For this review, take the finished solid that the model builds, in its own axes (mm). Face numbers are marked on the shaded views. Give positions to 0.01 mm unless a question says otherwise; leave off trailing zeros. Loops run counter-clockwise (first coordinate to the right, second up) from the corner with the lowest first, then second, coordinate; pieces in that order, holes last. Notation, with made-up numbers: (-3.75, -38) - (30.25, -38) arc R23 cw to (30.25, -9) - close; hole circle Ø10 at (44.25, 7). An arc over 180 degrees is marked (long way). Put each result on its own line as item: value. Start each with the question number.
from build123d import *

# Parameters (mm, degrees)
F2_R     = 2.9212519553
F3_DEPTH = 25


# Not quite as in the source:
# - a fillet or chamfer that OpenCascade refuses, or shapes differently, is made with other operations: its cross-section is extruded or revolved along the edge and cut away or added


with BuildPart() as f1:
    # F0 (on Front) → F1 (revolve)
    with BuildSketch(Plane.XZ):
        Polygon((0, 18.8674032688), (0, 15.0357997045), (10, 15.0357997045), (10, 18.8674032688), (6.7462138832, 18.8674032688), (6.7462138832, 29.4962655753), (17.0517656952, 29.4962655753), (17.0517656952, 34.9722243845), (0, 34.9722243845), (0, 29.4962655753), (2.411958063, 29.4962655753), (2.411958063, 18.8674032688), align=None)
    revolve(axis=Axis((6.3371746801, 0, 0), (1, 0, 0)))

    # F2 (on face) → F3 (cut)
    with BuildSketch(Plane(origin=(2.411958063, 0, 0), x_dir=(0, -1, 0), z_dir=(-1, 0, 0))):
        with Locations((-22.6866142127, 7.3713277985)):
            Circle(F2_R)
        with Locations((0, 23.8541178405)):
            Circle(F2_R)
        with Locations((22.6866142127, 7.3713277985)):
            Circle(F2_R)
        with Locations((14.0210986731, -19.2983867188)):
            Circle(F2_R)
        with Locations((-14.0210986731, -19.2983867188)):
            Circle(F2_R)
    extrude(amount=-F3_DEPTH, mode=Mode.SUBTRACT)

    # F4: fillet of radius 5 on 4 edges, made by hand

    # F4_s1 → F4_t2 (revolve, cut)
    with BuildSketch(Plane.XZ):
        with BuildLine():
            ThreePointArc((0, 29.9722243845), (1.4644660941, 33.5077582905), (5, 34.9722243845))
            Line((5, 34.9722243845), (5, 35.0722243845))
            Line((5, 35.0722243845), (-0.1, 35.0722243845))
            Line((-0.1, 35.0722243845), (-0.1, 29.9722243845))
            Line((-0.1, 29.9722243845), (0, 29.9722243845))
        make_face()
    revolve(axis=Axis((0, 0, 0), (1, 0, 0)), mode=Mode.SUBTRACT)

    # F4_s3 → F4_t4 (revolve, cut)
    with BuildSketch(Plane.XZ):
        with BuildLine():
            ThreePointArc((0, 18.8674032688), (1.7665712524, 16.1088427288), (4.8615686531, 15.0357997045))
            Line((4.8615686531, 15.0357997045), (4.8615686531, 14.9357997045))
            Line((4.8615686531, 14.9357997045), (0, 14.9357997045))
            Line((0, 14.9357997045), (-0.1, 15.0357997045))
            ThreePointArc((-0.1, 15.0357997045), (-0.1, 16.9516014867), (-0.0972313731, 18.8440353401))
            Line((-0.0972313731, 18.8440353401), (0, 18.8674032688))
        make_face()
    revolve(axis=Axis((0, 0, 0), (1, 0, 0)), mode=Mode.SUBTRACT)

    # F4_s5 → F4_t6 (revolve, cut)
    with BuildSketch(Plane.XZ):
        with BuildLine():
            ThreePointArc((12.0517656952, 34.9722243845), (15.5872996011, 33.5077582905), (17.0517656952, 29.9722243845))
            Line((17.0517656952, 29.9722243845), (17.1517656952, 29.9722243845))
            Line((17.1517656952, 29.9722243845), (17.1517656952, 35.0722243845))
            Line((17.1517656952, 35.0722243845), (12.0517656952, 35.0722243845))
            Line((12.0517656952, 35.0722243845), (12.0517656952, 34.9722243845))
        make_face()
    revolve(axis=Axis((17.0517656952, 0, 0), (1, 0, 0)), mode=Mode.SUBTRACT)

    # F4_s7 → F4_t8 (revolve, cut)
    with BuildSketch(Plane.XZ):
        with BuildLine():
            ThreePointArc((5.1384313469, 15.0357997045), (8.2334287476, 16.1088427288), (10, 18.8674032688))
            Line((10, 18.8674032688), (10.0972313731, 18.8440353401))
            ThreePointArc((10.0972313731, 18.8440353401), (10.1, 16.9516014867), (10.1, 15.0357997045))
            Line((10.1, 15.0357997045), (10, 14.9357997045))
            Line((10, 14.9357997045), (5.1384313469, 14.9357997045))
            Line((5.1384313469, 14.9357997045), (5.1384313469, 15.0357997045))
        make_face()
    revolve(axis=Axis((10, 0, 0), (1, 0, 0)), mode=Mode.SUBTRACT)


solid = f1.part
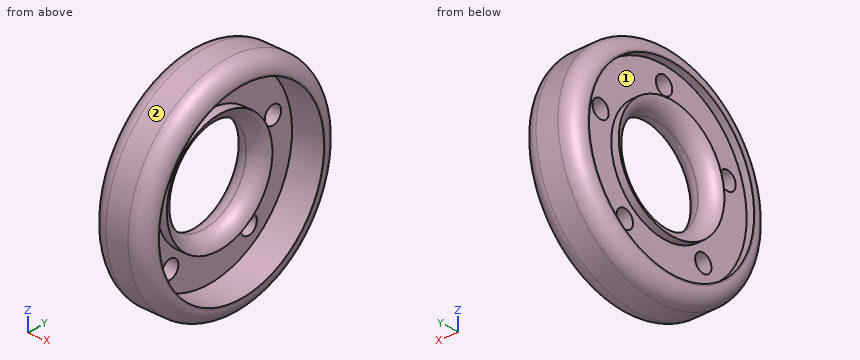
1) Mouldability with a two-part tool opening along Z and no side actions: class the marked faces 1 and 2 as released by +Z, released by -Z, zero draft, split by the parting line, or undercut.
2) Take a section at A-A on z = 0. State the section outline as (x, y) points.
3) Insertion check: P1, Ø24, axis at y = 0, z = 0, coming from the +X side; P2, Ø6.5, axis at y = -22.69, z = 7.37, coming from the -X side; P3, Ø4, axis at x = 3.5, z = -3, coming from the +Y side; P4, Ø10, axis at x = 14.5, z = 1, coming from the -Y side. Each pin has a flat end and moves straight along its axis. Give the tip position at first contact, or say it passes through.
4) Take a section at B-B on y = 0. State how many separate pieces and enclosed holes the cut face has, and give its area (3 significant figures).
5) Take a section at D-D on x = 8. State the section outline as (y, z) points, and give its area (3 significant figures).
6) Take a section at C-C on x = 3.25. State the section outline as (y, z) points.
7) Wall thickness on probe 1 along Z at (x, y) = (5.5, 0); probe 2 along Z at (x, y) = (11.75, 0); probe 3 along Z at (x, y) = (1.5, 3): over which ranges is each line inside the solid? List them lowest first.
Answers follow:
1. face 1: undercut
1. face 2: split by the parting line
2. outline: (0, -29.97) arc R5 ccw to (5, -34.97) - (12.05, -34.97) arc R5 ccw to (17.05, -29.97) - (17.05, -29.5) - (6.75, -29.5) - (6.75, -18.87) - (10, -18.87) arc R5 ccw to (5.14, -15.04) - (4.86, -15.04) arc R5 ccw to (0, -18.87) - (2.41, -18.87) - (2.41, -29.5) - (0, -29.5) - close; (0, 18.87) arc R5 ccw to (4.86, 15.04) - (5.14, 15.04) arc R5 ccw to (10, 18.87) - (6.75, 18.87) - (6.75, 29.5) - (17.05, 29.5) - (17.05, 29.97) arc R5 ccw to (12.05, 34.97) - (5, 34.97) arc R5 ccw to (0, 29.97) - (0, 29.5) - (2.41, 29.5) - (2.41, 18.87) - close
3. P1: through
3. P2: x = 2.41
3. P3: y = 34.94
3. P4: y = -34.97
4. separate pieces: 3
4. enclosed holes: 0
4. area: 290 mm2
5. outline: circle Ø69.94 at (0, 0); circle Ø37.73 at (0, 0); hole circle Ø58.99 at (0, 0); hole circle Ø31.87 at (0, 0)
5. area: 1,430 mm2
6. outline: circle Ø69.31 at (0, 0); hole circle Ø5.84 at (-22.69, 7.37); hole circle Ø5.84 at (-14.02, -19.3); hole circle Ø30.61 at (0, 0); hole circle Ø5.84 at (0, 23.85); hole circle Ø5.84 at (14.02, -19.3); hole circle Ø5.84 at (22.69, 7.37)
7. probe 1: -34.97 to -15.05, 15.05 to 20.93, 26.78 to 34.97
7. probe 2: -34.97 to -29.5, 29.5 to 34.97
7. probe 3: -33.41 to -29.34, -18.63 to -16.06, 16.06 to 18.63, 29.34 to 33.41
